Autodesk Inventor part; units mm, degrees
ref_plane "Start Plane" through (0, 0, -4.8828) normal (0, 0, 1) x (1, 0, 0)
ref_plane "End Plane" through (0, 0, 210.3644) normal (0, 0, 1) x (1, 0, 0)
ref_plane "Work Plane4" through (-9.8051, 4.2031, 221.3064) normal (0.7216, -0.3093, 0.6194) x (0.6785, 0.1378, -0.7216)
ref_plane "Start Plane" through (0, 0, -4.8828) normal (0, 0, 1) x (1, 0, 0)
ref_plane "End Plane" through (0, 0, 210.3644) normal (0, 0, 1) x (1, 0, 0)
sketch "Sketch" plane through (0, 0, 0) normal (0, 0, 1) x (1, 0, 0)
  circle A0 centre (0, 0) radius 6.9342
  circle A1 centre (0, 0) radius 10.668
  dimension "d0" = 21.336
  dimension "d1" = 3.7338
extrude "Body" add sketch "Sketch" along normal up to surface (215.2472 mm away) from surface at -4.8828
sketch "Sketch3" plane through (0, 0, 0) normal (0, 0, 1) x (1, 0, 0)
  line L0 (0, 0) -> (10, 0)
ref_plane "Work Plane3" through (0, 0, 0) normal (0, -1, 0) x (1, 0, 0)
sketch "Sketch4" plane through (0, 0, 0) normal (0, -1, 0) x (1, 0, 0)
  line L0 (-2, -4.8828) -> (12, -4.8828)
  line L1 (-2, 210.3644) -> (12, 210.3644)
  dimension "d7" = 215.2472
ref_plane "Work Plane4" through (-9.8051, 4.2031, 221.3064) normal (0.7216, -0.3093, 0.6194) x (0.6785, 0.1378, -0.7216)
split "Split1" plane through (-9.8051, 4.2031, 221.3064) removes the side toward (0.7216, -0.3093, 0.6194)
ref_plane "Work Plane5" through (6.7961, -8.2231, 217.0135) normal (-0.4168, 0.5043, 0.7563) x (0.9011, 0.1197, 0.4168)
split "Split2" plane through (6.7961, -8.2231, 217.0135) removes the side toward (-0.4168, 0.5043, 0.7563)
ref_plane "Work Plane6" through (-0.5919, -10.6516, -5.6452) normal (0.026, 0.467, -0.8839) x (0.9942, -0.1044, -0.026)
split "Split3" plane through (-0.5919, -10.6516, -5.6452) removes the side toward (0.026, 0.467, -0.8839)
ref_plane "Work Plane7" through (-10.6583, -0.4551, -8.3573) normal (0.6161, 0.0263, -0.7872) x (-0.7839, -0.0762, -0.6161)
split "Split4" plane through (-10.6583, -0.4551, -8.3573) removes the side toward (0.6161, 0.0263, -0.7872)
ref_plane "Work Plane8" through (3.7346, -9.993, -10.2024) normal (-0.242, 0.6474, -0.7227) x (0.7889, 0.5649, 0.242)
split "Split5" plane through (3.7346, -9.993, -10.2024) removes the side toward (-0.242, 0.6474, -0.7227)
equation "\"d0\" = G_H"
equation "\"d1\" = G_T"
equation "\"d2\" = G_L"
equation "\"G_H\" = 21.336"
equation "\"G_T\" = 3.7338"
equation "\"G_L\" = 215.24718"
equation "\"G_OFFSET_START\" = 4.88279"
equation "\"G_OFFSET_END\" = 2.57893"
equation "\"d4\" = -G_OFFSET_START"
equation "\"d5\" = G_OFFSET_END + B_L"
equation "\"B_L\" = 207.78546"
properties part number "ANSI - 1/2 x 0.147 - 8.474" material "Steel, Mild"
For this review, take the finished solid that the model builds, in its own axes (mm). Coordinates: 2 decimals unless noted, no trailing zeros. Write each loop counter-clockwise with the first axis right and the second up, starting at its lowest first coordinate (ties: lowest second). Pieces come first, ordered by that corner, then holes. Notation, with made-up numbers: (19, 75.25) - (46, 75.25) arc R13 cw to (46, 91.25) - close; hole circle Ø3 at (53.5, -32.75). An arc over 180 degrees is marked (long way). Answer in a Markdown table with one row per item. Add a question column.
Q1. For P1, Ø12, axis at y = -7, z = 36, coming from the +X side; P2, Ø1, axis at x = -6, z = 39, coming from the -Y side; P3, Ø12, axis at x = -7.5, y = 2.5, coming from the +Z side, all flat-tipped, find the tip position at first contact; note any pin that passes through.
Q2. Draft analysis for pull direction Y (two halves, no side actions). For faces 1 (the cylindrical face through (6.614, -2.083, 101.655)), 2 (the flat face through (4.766, -5.305, 199.583)), 3 (the cylindrical face through (-7.86, -7.21, 101.23)), 4 (the flat face through (-6.7, 3.5, 201.76)), state which applies: +Y half, -Y half, draft (parallel to the pull), parting line (faces both ways), or undercut.
Q3. We need section C-C, the plane x = 0.25. State the section outline as (y, z) points.
Q4. We need section A-A, the plane y = -2.75. State the section outline as (x, z) points, and give its area (3 significant figures).
Q5. We need section B-B, the plane z = 67. State the section outline as (x, y) points, and give its area (3 significant figures).
Q6. For probe 1 along Y at (x, z) = (0, 71.5); probe 2 along X at (y, z) = (3.25, 110), list the stretches that pass through material, from the lowest coordinate up.
Answer list:
| question | item | result |
|---|---|---|
| 1 | P1 | stops at x = 10.62 |
| 1 | P2 | stops at y = -9.14 |
| 1 | P3 | stops at z = 206.65 |
| 2 | face 1 | undercut |
| 2 | face 2 | -Y half |
| 2 | face 3 | parting line |
| 2 | face 4 | +Y half |
| 3 | outline | (-10.67, -0.16) - (-6.93, -0.04) - (-6.93, 204.03) - (-10.67, 202.17) - close; (6.93, 6.12) - (10.67, 9.47) - (10.67, 200.81) - (6.93, 203.3) - close |
| 4 | outline | (-10.31, 0.99) - (-6.37, -0.33) - (-6.37, 206.11) - (-10.31, 203.94) - close; (6.37, 4.89) - (10.31, 7.97) - (10.31, 194.4) - (6.37, 199) - close |
| 4 | area | 1,560 mm2 |
| 5 | outline | circle Ø21.34 at (0, 0); hole circle Ø13.87 at (0, 0) |
| 5 | area | 206 mm2 |
| 6 | probe 1 | y = -10.67 to -6.93, 6.93 to 10.67 |
| 6 | probe 2 | x = -10.16 to -6.13, 6.13 to 10.16 |
